```python
from build123d import *

# Parameters (mm, degrees)
SKETCH1_W             = 25.4
SKETCH1_H             = 25.4
SKETCH1_W_2           = 19.05
SKETCH1_H_2           = 19.05
BOSS_EXTRUDE1_DEPTH   = 292.1
SKETCH3_W             = 2.4892
SKETCH3_H             = 25.4
SKETCH3_AT_POINT_2_W  = 2.4892
SKETCH3_AT_POINT_2_H  = 25.4
LPATTERN1_START       = -12.7
LPATTERN1_OUTLINE_R   = 2.4892
LPATTERN1_DEPTH       = 25.4
LPATTERN1_2_OUTLINE_R = 2.4892
LPATTERN1_2_DEPTH     = 25.4


# Read off the part's stored shape, not the designer's step: LPattern1
with BuildPart() as part:
    # Sketch1 → Boss-Extrude1 (new, symmetric)
    with BuildSketch(Plane(origin=(0, 0, 0), x_dir=(0, 0, -1), z_dir=(1, 0, 0))):
        Rectangle(SKETCH1_W, SKETCH1_H)
        Rectangle(SKETCH1_W_2, SKETCH1_H_2, mode=Mode.SUBTRACT)
    extrude(amount=BOSS_EXTRUDE1_DEPTH, both=True)

    # Sketch3 → #9 (0.196) Diameter Hole1 (revolve, cut)
    with BuildSketch(Plane(origin=(279.4, 12.7, 0), x_dir=(0, 0, 1), z_dir=(1, 0, 0))):
        with Locations((1.2446, 12.7)):
            Rectangle(SKETCH3_W, SKETCH3_H)
    revolve(axis=Axis((279.4, 19.05, 0), (0, -1, 0)), mode=Mode.SUBTRACT)

    # Sketch3 at point 2 (carried to point 2, square into its face) → #9 (0.196) Diameter Hole1 at 2 (revolve, cut)
    with BuildSketch(Plane(origin=(279.400011186, 0.016856195, 12.7), x_dir=(0, -1, 0), z_dir=(1, 0, 0))):
        with Locations((1.2446, 12.7)):
            Rectangle(SKETCH3_AT_POINT_2_W, SKETCH3_AT_POINT_2_H)
    revolve(axis=Axis((279.400011186, 0.016856195, 19.05), (0, 0, -1)), mode=Mode.SUBTRACT)

    # LPattern1 outline → LPattern1 (cut)
    with BuildSketch(Plane.XY.offset(LPATTERN1_START)):
        with Locations((254.000011186, 0.016856195)):
            Circle(LPATTERN1_OUTLINE_R)
        with Locations((228.600011186, 0.016856195)):
            Circle(LPATTERN1_OUTLINE_R)
        with Locations((203.200011186, 0.016856195)):
            Circle(LPATTERN1_OUTLINE_R)
        with Locations((177.800011186, 0.016856195)):
            Circle(LPATTERN1_OUTLINE_R)
        with Locations((152.400011186, 0.016856195)):
            Circle(LPATTERN1_OUTLINE_R)
        with Locations((127.000011186, 0.016856195)):
            Circle(LPATTERN1_OUTLINE_R)
        with Locations((101.600011186, 0.016856195)):
            Circle(LPATTERN1_OUTLINE_R)
        with Locations((76.200011186, 0.016856195)):
            Circle(LPATTERN1_OUTLINE_R)
        with Locations((50.800011186, 0.016856195)):
            Circle(LPATTERN1_OUTLINE_R)
        with Locations((25.400011186, 0.016856195)):
            Circle(LPATTERN1_OUTLINE_R)
        with Locations((1.1186e-05, 0.016856195)):
            Circle(LPATTERN1_OUTLINE_R)
        with Locations((-25.399988814, 0.016856195)):
            Circle(LPATTERN1_OUTLINE_R)
        with Locations((-50.799988814, 0.016856195)):
            Circle(LPATTERN1_OUTLINE_R)
        with Locations((-76.199988814, 0.016856195)):
            Circle(LPATTERN1_OUTLINE_R)
        with Locations((-101.599988814, 0.016856195)):
            Circle(LPATTERN1_OUTLINE_R)
        with Locations((-126.999988814, 0.016856195)):
            Circle(LPATTERN1_OUTLINE_R)
        with Locations((-152.399988814, 0.016856195)):
            Circle(LPATTERN1_OUTLINE_R)
        with Locations((-177.799988814, 0.016856195)):
            Circle(LPATTERN1_OUTLINE_R)
        with Locations((-203.199988814, 0.016856195)):
            Circle(LPATTERN1_OUTLINE_R)
        with Locations((-228.599988814, 0.016856195)):
            Circle(LPATTERN1_OUTLINE_R)
        with Locations((-253.999988814, 0.016856195)):
            Circle(LPATTERN1_OUTLINE_R)
        with Locations((-279.399988814, 0.016856195)):
            Circle(LPATTERN1_OUTLINE_R)
    extrude(amount=LPATTERN1_DEPTH, mode=Mode.SUBTRACT)

    # LPattern1 2 outline → LPattern1 2 (cut)
    with BuildSketch(Plane(origin=(0, 0, 0), x_dir=(1, 0, 0), z_dir=(0, 1, 0)).offset(LPATTERN1_START)):
        with Locations((254, 0)):
            Circle(LPATTERN1_2_OUTLINE_R)
        with Locations((228.6, 0)):
            Circle(LPATTERN1_2_OUTLINE_R)
        with Locations((203.2, 0)):
            Circle(LPATTERN1_2_OUTLINE_R)
        with Locations((177.8, 0)):
            Circle(LPATTERN1_2_OUTLINE_R)
        with Locations((152.4, 0)):
            Circle(LPATTERN1_2_OUTLINE_R)
        with Locations((127, 0)):
            Circle(LPATTERN1_2_OUTLINE_R)
        with Locations((101.6, 0)):
            Circle(LPATTERN1_2_OUTLINE_R)
        with Locations((76.2, 0)):
            Circle(LPATTERN1_2_OUTLINE_R)
        with Locations((50.8, 0)):
            Circle(LPATTERN1_2_OUTLINE_R)
        with Locations((25.4, 0)):
            Circle(LPATTERN1_2_OUTLINE_R)
        Circle(LPATTERN1_2_OUTLINE_R)
        with Locations((-25.4, 0)):
            Circle(LPATTERN1_2_OUTLINE_R)
        with Locations((-50.8, 0)):
            Circle(LPATTERN1_2_OUTLINE_R)
        with Locations((-76.2, 0)):
            Circle(LPATTERN1_2_OUTLINE_R)
        with Locations((-101.6, 0)):
            Circle(LPATTERN1_2_OUTLINE_R)
        with Locations((-127, 0)):
            Circle(LPATTERN1_2_OUTLINE_R)
        with Locations((-152.4, 0)):
            Circle(LPATTERN1_2_OUTLINE_R)
        with Locations((-177.8, 0)):
            Circle(LPATTERN1_2_OUTLINE_R)
        with Locations((-203.2, 0)):
            Circle(LPATTERN1_2_OUTLINE_R)
        with Locations((-228.6, 0)):
            Circle(LPATTERN1_2_OUTLINE_R)
        with Locations((-254, 0)):
            Circle(LPATTERN1_2_OUTLINE_R)
        with Locations((-279.4, 0)):
            Circle(LPATTERN1_2_OUTLINE_R)
    extrude(amount=LPATTERN1_2_DEPTH, mode=Mode.SUBTRACT)


solid = part.part
```
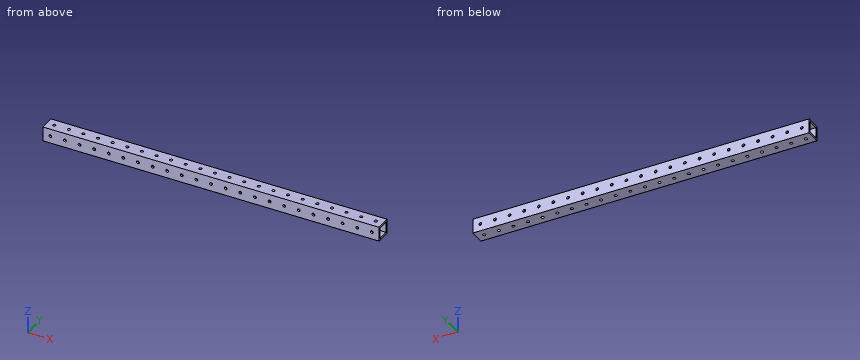
Verification items for the finished model (mm, model axes). Give positions to 0.01 mm unless a question says otherwise; leave off trailing zeros. Loops run counter-clockwise (first coordinate to the right, second up) from the corner with the lowest first, then second, coordinate; pieces in that order, holes last.
1. Go/stop test with a flat-tipped pin: pin 1 Ø3 at (x, y) = (-152.4, 0.02) entering from +Z. Record where the tip stops, or that it passes through.
2. Thickness scan on line 1 (Z direction, x = 239, y = -8.75) (3 decimals); line 2 (Z direction, x = -101.6, y = -11.1). Record the ranges inside material, lowest first.
3. Section check A-A, the plane x = -162.5. Enter the section's corners in (y, z) (3 decimals), then the cut area to 3 significant figures.
Geometry says:
1. pin 1: passes through
2. line 1: z = -12.7 to -9.525, 9.525 to 12.7
2. line 2: z = -12.7 to -2.49, 2.49 to 12.7
3. outline: (-12.7, -12.7) - (12.7, -12.7) - (12.7, 12.7) - (-12.7, 12.7) - close; hole (-9.525, -9.525) - (9.525, -9.525) - (9.525, 9.525) - (-9.525, 9.525) - close
3. area: 282 mm2
